from build123d import *

# Parameters (mm, degrees)
SKETCH1_R           = 7.55
SKETCH1_R_2         = 5
SKETCH1_R_3         = 10.55
BOSS_EXTRUDE1_DEPTH = 10
SKETCH4_R           = 7.5
BOSS_EXTRUDE2_DEPTH = 30
BOSS_EXTRUDE2_TAPER = 7
SKETCH5_R           = 1.25
CUT_EXTRUDE2_DEPTH  = 10
FILLET1_R           = 15
FILLET2_R           = 7.5


with BuildPart() as part:
    # Sketch1 → Boss-Extrude1 (new body)
    with BuildSketch(Plane(origin=(0, 0, 0), x_dir=(1, 0, 0), z_dir=(0, 1, 0))):
        Polygon((23.995878661, -35), (56.995878661, -35), (56.995878661, -75), (88.995878661, -75), (88.995878661, -25), (88.995878661, 25), (17.5, 25), (-2.004121339, 25), (-2.004121339, 7.840472806), (23.995878661, 7.840472806), (23.995878661, 0), align=None)
        with Locations((73.995878661, 0)):
            Circle(SKETCH1_R, mode=Mode.SUBTRACT)
        with Locations((51.495878661, 0)):
            Circle(SKETCH1_R_2, mode=Mode.SUBTRACT)
        with Locations((73.995878661, -60)):
            Circle(SKETCH1_R_3, mode=Mode.SUBTRACT)
    extrude(amount=BOSS_EXTRUDE1_DEPTH)

    # Sketch4 → Boss-Extrude2 (add)
    with BuildSketch(Plane(origin=(0, 10, 0), x_dir=(1, 0, 0), z_dir=(0, 1, 0))):
        with Locations((6.495878661, 16.5)):
            Circle(SKETCH4_R)
    extrude(amount=BOSS_EXTRUDE2_DEPTH, taper=BOSS_EXTRUDE2_TAPER)

    # Sketch5 → Cut-Extrude2 (cut)
    with BuildSketch(Plane(origin=(0, 40, 0), x_dir=(1, 0, 0), z_dir=(0, 1, 0))):
        with Locations((6.495878661, 16.5)):
            Circle(SKETCH5_R)
    extrude(amount=-CUT_EXTRUDE2_DEPTH, mode=Mode.SUBTRACT)

    # Fillet1
    fillet1_edges = [part.edges().sort_by_distance(p)[0] for p in [
        (88.995878661, 5, -25),
        (88.995878661, 5, 75),
        (56.995878661, 5, 75),
        (23.995878661, 5, 35),
        (23.995878661, 5, -7.840472806),
    ]]
    fillet(fillet1_edges, radius=FILLET1_R)

    # Fillet2
    fillet2_edges = [part.edges().sort_by_distance(p)[0] for p in [
        (-2.004121339, 5, -7.840472806),
        (-2.004121339, 5, -25),
    ]]
    fillet(fillet2_edges, radius=FILLET2_R)


solid = part.part
Read the model definition and answer for the solid it produces. Units are mm, in the model's axes. A direction names the side the tool comes from. Give positions to 0.01 mm unless a question says otherwise; leave off trailing zeros. Write each loop counter-clockwise with the first axis right and the second up, starting at its lowest first coordinate (ties: lowest second). Pieces come first, ordered by that corner, then holes. Notation, with made-up numbers: (29.25, 12) -> (63.25, 12) arc R27 cw to (63.25, 36) -> close; hole circle Ø11 at (47.5, 41.25). An arc over 180 degrees is marked (long way). Answer as a JSON object with one key per item and string values. Group by question number.
1) The mould has two halves that part along Z. Classify faces 1 (the flat face through (-2.004, 5, -16)), 2 (the conical face through (2.03, 25.21, -13.07)), 3 (the cylindrical face through (46.5, 4.9, -0.2)): +Z half, -Z half, draft (parallel to the pull), parting line (faces both ways), or undercut.
2) Find section D-D (y = 32.5). Write down the section's boundary in (x, z), and give its area (3 significant figures).
3) A tool of negligible diameter and unlimited length cuts with its end or side. For faces 4 (the flat face through (7, 5, -7.84)), 5 (the cylindrical face through (5.57, 35.07, -17.34)), 6 (the cylindrical face through (84.49, 5.07, 70.72)), from which of +Z, -Z, +X, -X, +Y, -Y can it reach the whole face along a straight path? Write none if from no direction.
4) Find section A-A (z = 0). Write down the section's boundary in (x, y), and give its area (3 significant figures).
5) Find section C-C (z = 17). Write down the section's boundary in (x, y), and give its area (3 significant figures).
6) Find section B-B (x = 49.5). Write down the section's boundary in (y, z), and give its area (3 significant figures).
7) Each of these flat-tipped pins is pushed along its axis until it touches: P1, Ø8, axis at x = 68, z = 40.5, coming from the +Y side; P2, Ø5, axis at x = 44.5, z = 29, coming from the -Y side; P3, Ø5, axis at y = 7, z = 12, coming from the -X side; P4, Ø19, axis at x = 74, z = 60, coming from the +Y side. Where does it stop, or does it pass through?
8) Consider L1, parallel to X at y = 8, z = 60; L2, parallel to X at y = 2, z = 0; L3, parallel to Y at x = 36, z = 14.5. Determine where each line is inside the solid, lowest interval first. Write a range as from..to.
Values follow:
{
 "1": {"face 1": "draft", "face 2": "parting line", "face 3": "undercut"},
 "2": {"outline": "circle Ø9.47 at (6.5, -16.5); hole circle Ø2.5 at (6.5, -16.5)", "area": "65.6 mm2"},
 "3": {"face 4": "+Z, -X, +Y, -Y", "face 5": "+Y", "face 6": "+Z, +X, +Y, -Y"},
 "4": {"outline": "(22.18, 0) -> (46.5, 0) -> (46.5, 10) -> (22.18, 10) -> close; (56.5, 0) -> (66.45, 0) -> (66.45, 10) -> (56.5, 10) -> close; (81.55, 0) -> (89, 0) -> (89, 10) -> (81.55, 10) -> close", "area": "417 mm2"},
 "5": {"outline": "(24, 0) -> (89, 0) -> (89, 10) -> (24, 10) -> close", "area": "650 mm2"},
 "6": {"outline": "(0, -25) -> (10, -25) -> (10, -4.58) -> (0, -4.58) -> close; (0, 4.58) -> (10, 4.58) -> (10, 35) -> (0, 35) -> close", "area": "508 mm2"},
 "7": {"P1": "stops at y = 10", "P2": "stops at y = 0", "P3": "stops at x = 24", "P4": "passes through"},
 "8": {"L1": "x = 57..63.45, 84.55..89", "L2": "x = 22.18..46.5, 56.5..66.45, 81.55..89", "L3": "y = 0..10"}
}
